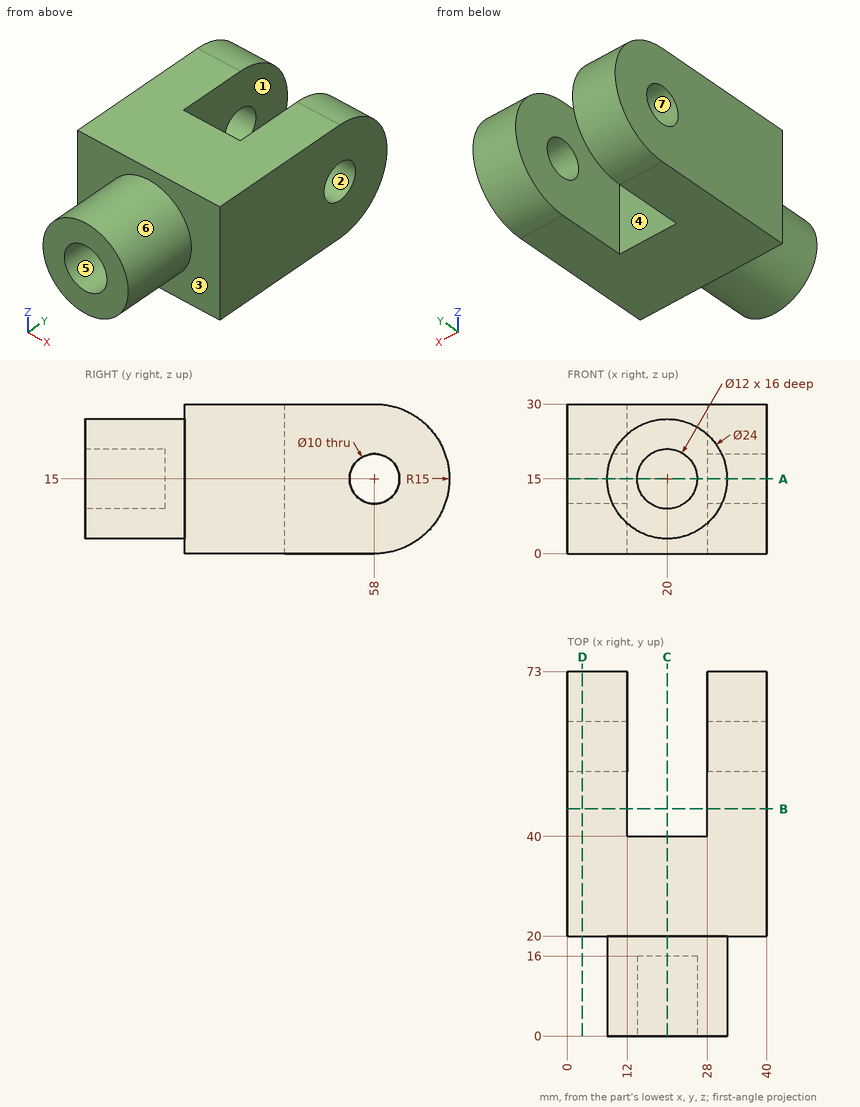
Source: three-view drawing plus pictorial views. Frame: mm from the lowest corner of the part. A direction names the side the tool comes from. Round coordinates to 2 decimals unless told otherwise and drop trailing zeros. Loops run counter-clockwise (first coordinate to the right, second up) from the corner with the lowest first, then second, coordinate; pieces in that order, holes last.
Q1. Access query for the marked faces 1, 2 and 3. Directions: +Z, -Z, +X, -X, +Y, -Y. A direction counts if a zero-diameter tool reaches every point of the face in a straight line with its end or side. Return the directions, or none.
Q2. Section B-B on y = 45.5. Return loops of the section in (x, z), plus the area to 3 significant figures.
Q3. Section C-C on x = 20. Return loops of the section in (y, z).
Q4. Pin query (flat end, axial travel): P1, Ø4, axis at x = 29, y = 16, coming from the -Z side; P2, Ø8, axis at x = 21, z = 12.5, coming from the +Y side; P3, Ø6, axis at x = 19, z = 17.5, coming from the -Y side; P4, Ø9, axis at y = 61, z = 14, coming from the -X side. Return the tip coordinate at first contact, or that it passes through.
Q5. Section D-D on x = 3. Return loops of the section in (y, z), plus the area to 3 significant figures.
Q6. Section A-A on z = 15. Return loops of the section in (x, y).
Q7. Pull-direction query (X, two-part tool) for the marked faces 4, 5, 6 and 7; classes: released by +X, released by -X, zero draft, split by the parting line, or undercut.
Q8. Material intervals for L1, parallel to Z at x = 8.5, y = 58; L2, parallel to Y at x = 37, z = 15.25; L3, parallel to X at y = 60.5, z = 21.5, sorted ascending.
Evaluation:
1. face 1: +Z, -Z, +Y
1. face 2: +X, -X
1. face 3: -Y
2. outline: (0, 0) - (12, 0) - (12, 30) - (0, 30) - close; (28, 0) - (40, 0) - (40, 30) - (28, 30) - close
2. area: 720 mm2
3. outline: (0, 3) - (20, 3) - (20, 0) - (40, 0) - (40, 30) - (20, 30) - (20, 27) - (0, 27) - (0, 21) - (16, 21) - (16, 9) - (0, 9) - close
4. P1: stops at z = 5.25
4. P2: stops at y = 40
4. P3: stops at y = 16
4. P4: stops at x = 0
5. outline: (20, 0) - (58, 0) arc R15 ccw to (58, 30) - (20, 30) - close; hole circle Ø10 at (58, 15)
5. area: 1,410 mm2
6. outline: (0, 20) - (8, 20) - (8, 0) - (14, 0) - (14, 16) - (26, 16) - (26, 0) - (32, 0) - (32, 20) - (40, 20) - (40, 53) - (28, 53) - (28, 40) - (12, 40) - (12, 53) - (0, 53) - close; (0, 63) - (12, 63) - (12, 73) - (0, 73) - close; (28, 63) - (40, 63) - (40, 73) - (28, 73) - close
7. face 4: undercut
7. face 5: undercut
7. face 6: split by the parting line
7. face 7: zero draft
8. L1: z = 0 to 10, 20 to 30
8. L2: y = 20 to 53.01, 62.99 to 73
8. L3: x = 0 to 12, 28 to 40
